Design review of the part built by this model. Coordinates are the model's own, in mm. Face numbers are marked on the shaded views. A direction names the side the tool comes from. Coordinates: 2 decimals unless noted, no trailing zeros. Order: outer loops, then holes, each group sorted by start corner. A loop starts at its lowest first (then second) coordinate and runs counter-clockwise, first axis right, second up. Notation, with made-up numbers: M 2,10 L 32,10 A18 ccw 32,21 Z; hole C 2,-10 d4. An arc over 180 degrees is marked long. Answer in a Markdown table with one row per item.
from build123d import *

# Parameters (mm, degrees)
F0_R     = 3.175
F1_DEPTH = 6.35


with BuildPart() as f1:
    # F0 (on Top) → F1 (new body)
    with BuildSketch(Plane.XY):
        with BuildLine():
            Line((31.75, -16.951759), (31.75, 16.951759))
            Line((31.75, 16.951759), (9.525, 16.951759))
            ThreePointArc((9.525, 16.951759), (0, 7.426759), (-9.525, 16.951759))
            Line((-9.525, 16.951759), (-31.75, 16.951759))
            Line((-31.75, 16.951759), (-31.75, -16.951759))
            Line((-31.75, -16.951759), (-19.05, -16.951759))
            Line((-19.05, -16.951759), (-19.05, -10.601759))
            Line((-19.05, -10.601759), (19.05, -10.601759))
            Line((19.05, -10.601759), (19.05, -16.951759))
            Line((19.05, -16.951759), (31.75, -16.951759))
        make_face()
        with Locations((-14.9987, 1.953059)):
            Circle(F0_R, mode=Mode.SUBTRACT)
        with Locations((14.9987, 1.953059)):
            Circle(F0_R, mode=Mode.SUBTRACT)
        with BuildLine():
            Line((9.525, 16.951759), (31.75, 16.951759))
            ThreePointArc((31.75, 16.951759), (0, 48.701759), (-31.75, 16.951759))
            Line((-31.75, 16.951759), (-9.525, 16.951759))
            ThreePointArc((-9.525, 16.951759), (0, 26.476759), (9.525, 16.951759))
        make_face()
        with Locations((-14.9987, 31.950459)):
            Circle(F0_R, mode=Mode.SUBTRACT)
        with Locations((14.9987, 31.950459)):
            Circle(F0_R, mode=Mode.SUBTRACT)
    extrude(amount=F1_DEPTH)


solid = f1.part
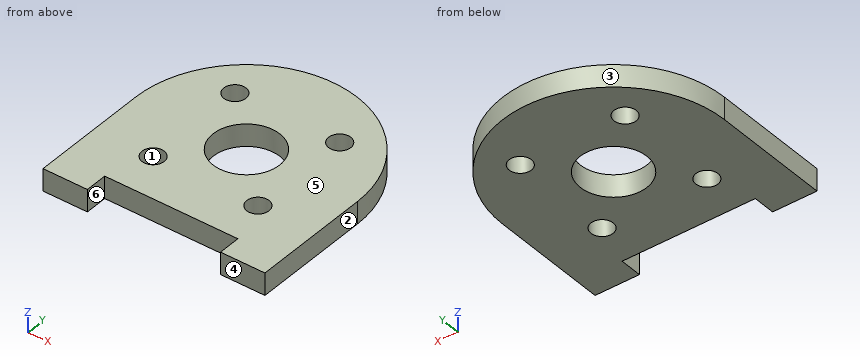
(1) For the marked faces 5 and 6, list the 3-axis set-ups (+Z, -Z, +X, -X, +Y, -Y) from which the entire face can be reached by the end or side of a thin tool; tool diameter is ignored.
Return value:
| item | result |
|---|---|
| face 5 | +Z, +X, -X, +Y, -Y |
| face 6 | +Z, -Z, -Y |
(2) Add section A-A, the plane x = 0. Give the boundary of the cut face in (y, z), and give its area (3 significant figures).
Return value:
| item | result |
|---|---|
| outline | M -10.6,0 L 7.43,0 L 7.43,6.35 L -10.6,6.35 Z; M 26.48,0 L 48.7,0 L 48.7,6.35 L 26.48,6.35 Z |
| area | 256 mm2 |
(3) For line 1 along X through (y, z) = (16.5, 3); line 2 along Y through (x, z) = (15.5, 4.5); line 3 along X through (y, z) = (31.5, 1), list the stretches that pass through material, from the lowest coordinate up. Write a range as from..to.
Return value:
| item | result |
|---|---|
| line 1 | x = -31.75..-9.51, 9.51..31.75 |
| line 2 | y = -10.6..-1.18, 5.09..28.82, 35.09..44.66 |
| line 3 | x = -28.22..-18.14, -11.86..11.86, 18.14..28.22 |
(4) Add section C-C, the plane x = -16. Give the boundary of the cut face in (y, z).
Return value:
| item | result |
|---|---|
| outline | M -10.6,0 L -1.06,0 L -1.06,6.35 L -10.6,6.35 Z; M 4.97,0 L 28.94,0 L 28.94,6.35 L 4.97,6.35 Z; M 34.96,0 L 44.38,0 L 44.38,6.35 L 34.96,6.35 Z |
(5) Add section D-D, the plane z = 3.5. Give the boundary of the cut face in (x, y) (3 decimals).
Return value:
| item | result |
|---|---|
| outline | M -31.75,-16.952 L -19.05,-16.952 L -19.05,-10.602 L 19.05,-10.602 L 19.05,-16.952 L 31.75,-16.952 L 31.75,16.952 A31.75 ccw -31.75,16.952 Z; hole C -14.999,1.953 d6.35; hole C -14.999,31.95 d6.35; hole C 0,16.952 d19.05; hole C 14.999,1.953 d6.35; hole C 14.999,31.95 d6.35 |
(6) Insertion check: pin 1 Ø1.9 at (x, z) = (-4.5, 3) entering from -Y; pin 2 Ø3 at (y, z) = (28, 2.5) entering from -X. Each pin has a flat end and moves straight along its axis. Give the tip position at first contact, or say it passes through.
Return value:
| item | result |
|---|---|
| pin 1 | stops at y = -10.6 |
| pin 2 | stops at x = -30.28 |
(7) Draft analysis for pull direction Y (two halves, no side actions). For the marked faces 1, 2, 3 and 4, state which applies: pulls with the +Y half, pulls with the -Y half, needs draft (parallel to the pull), parting line crosses it, or undercut.
Return value:
| item | result |
|---|---|
| face 1 | undercut |
| face 2 | needs draft |
| face 3 | pulls with the +Y half |
| face 4 | pulls with the -Y half |
(8) Add section B-B, the plane y = 16. Give the boundary of the cut face in (x, z).
Return value:
| item | result |
|---|---|
| outline | M -31.75,0 L -9.48,0 L -9.48,6.35 L -31.75,6.35 Z; M 9.48,0 L 31.75,0 L 31.75,6.35 L 9.48,6.35 Z |
